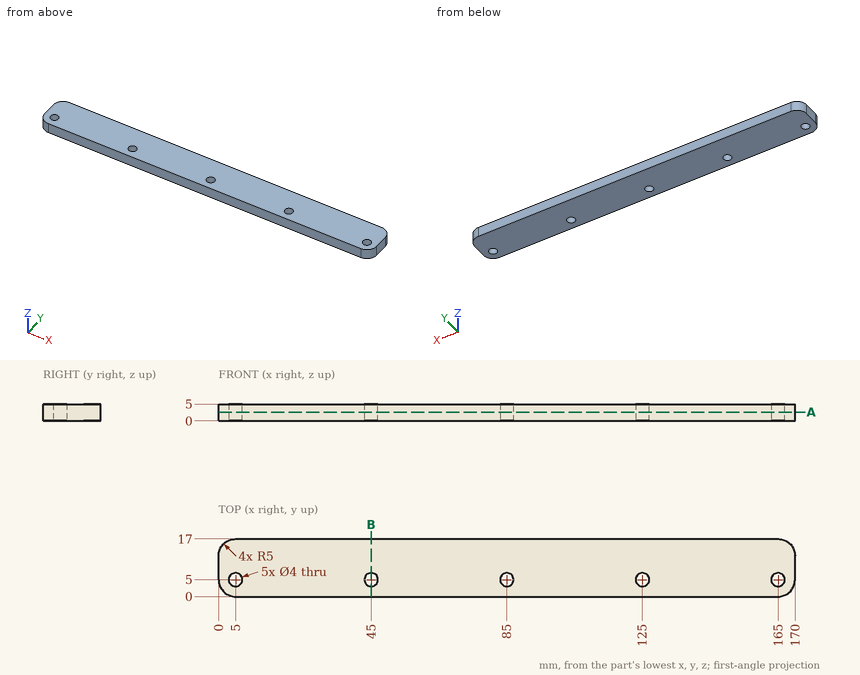
The figure shows three views and two pictorial views of one solid part (mm, origin at its lowest corner). Answer the questions. Coordinates: 2 decimals unless noted, no trailing zeros. Loops run counter-clockwise (first coordinate to the right, second up) from the corner with the lowest first, then second, coordinate; pieces in that order, holes last. Notation, with made-up numbers: (72, 5.5) -> (76, 5.5) arc R25 cw to (76, 43.5) -> close; hole circle Ø4 at (45.5, 62.25). An arc over 180 degrees is marked (long way). Return JSON: item names as keys, results as strings. Group by question number.
(1) A cutting plane is placed at A-A on z = 2.6. Write down the section's boundary in (x, y).
(2) Find the intervals of material crossed by probe 1 along Y at (x, z) = (165, 3.3); probe 2 along X at (y, z) = (6.5, 0.6); probe 3 along X at (y, z) = (13, 2.55), in increasing order. Write a range as from..to.
(3) Given pin 1 Ø5 at (x, y) = (125, 5) entering from -Z; pin 2 Ø2.5 at (x, y) = (165, 5) entering from +Z, each flat-ended and moving along its own axis, determine where each tip first touches the part or whether it passes through.
(4) A cutting plane is placed at B-B on x = 45. Write down the section's boundary in (y, z), and give its area (3 significant figures).
The answers:
{
 "1": {"outline": "(0, 5) arc R5 ccw to (5, 0) -> (165, 0) arc R5 ccw to (170, 5) -> (170, 12) arc R5 ccw to (165, 17) -> (5, 17) arc R5 ccw to (0, 12) -> close; hole circle Ø4 at (5, 5); hole circle Ø4 at (45, 5); hole circle Ø4 at (85, 5); hole circle Ø4 at (125, 5); hole circle Ø4 at (165, 5)"},
 "2": {"probe 1": "y = 0..3, 7..17", "probe 2": "x = 0..3.68, 6.32..43.68, 46.32..83.68, 86.32..123.68, 126.32..163.68, 166.32..170", "probe 3": "x = 0.1..169.9"},
 "3": {"pin 1": "stops at z = 0", "pin 2": "passes through"},
 "4": {"outline": "(0, 0) -> (3, 0) -> (3, 5) -> (0, 5) -> close; (7, 0) -> (17, 0) -> (17, 5) -> (7, 5) -> close", "area": "65.0 mm^2"}
}
